Verification items for the finished model (mm, model axes). A direction names the side the tool comes from. Coordinates: 2 decimals unless noted, no trailing zeros. Order: outer loops, then holes, each group sorted by start corner. A loop starts at its lowest first (then second) coordinate and runs counter-clockwise, first axis right, second up. Notation, with made-up numbers: M 43.5,42 L 50.5,42 A8 ccw 50.5,51 Z; hole C 52.5,-11.5 d5. An arc over 180 degrees is marked long. Answer as a JSON object with one key per item and string values. Group by question number.
(1) Cross-section at A-A (z = 0). Count the separate pieces of the cut face and the enclosed holes in it, plus the area to 3 significant figures.
(2) Mould release check, pull along Z, two halves, no side actions. Record for faces 6 (the face through (1.99, -57.15, 0.84)), 7 (the face through (0, -22, 16)), 8 (the face through (2.15, 0.84, -56.99)): released by +Z, released by -Z, zero draft, split by the parting line, or undercut.
(3) Gauge pin test, flat ends, axial feed: pin 1 Ø3 at (x, y) = (-10.5, -2) entering from +Z; pin 2 Ø10 at (x, z) = (-11, -3.5) entering from +Y; pin 3 Ø3 at (x, y) = (-1.5, 25) entering from +Z; pin 4 Ø2 at (x, z) = (-4, -9) entering from -Y. Record the tip position at first contact, or that the pin passes through.
(4) Cross-section at C-C (x = -21.5). Enter the section's corners in (y, z), plus the area to 3 significant figures.
(5) Material ranges on line 1 (X direction, y = 31, z = -15); line 2 (Y direction, x = -4.5, z = -39); line 3 (Z direction, x = -1.75, y = 25), recorded low to high.
(6) Access from +Z, -Z, +X, -X, +Y, -Y to the whole of each face (thin tool, end or side, straight path). Record for faces 1 (the face through (-15, 28.333, 0)), 2 (the face through (-10, 0, 10)), 3 (the face through (0, 22, -16)), 4 (the face through (0, 29.333, 0)), 5 (the face through (-10, 0, -10)).
from build123d import *

# Parameters (mm, degrees)
SKETCH2_W           = 120
SKETCH2_H           = 120
BOSS_EXTRUDE1_DEPTH = 5
FILLET1_R           = 10
BOSS_EXTRUDE2_DEPTH = 50
SKETCH3_W           = 12.5
SKETCH3_H           = 30
CUT_EXTRUDE1_DEPTH  = 91
SKETCH5_W           = 14.5
SKETCH5_H           = 32
CUT_EXTRUDE2_DEPTH  = 10


with BuildPart() as part:
    # Sketch2 → Boss-Extrude1 (new, symmetric)
    with BuildSketch(Plane.YZ):
        Rectangle(SKETCH2_W, SKETCH2_H)
    extrude(amount=BOSS_EXTRUDE1_DEPTH, both=True)

    # Fillet1
    fillet1_edges = [part.edges().sort_by_distance(p)[0] for p in [
        (5, 60, 0),
        (5, 0, -60),
        (5, -60, 0),
        (5, 0, 60),
    ]]
    fillet(fillet1_edges, radius=FILLET1_R - 0.0001)  # a hair under: the kernel refuses the full size

    # Sketch4 → Boss-Extrude2 (add, symmetric)
    with BuildSketch(Plane(origin=(0, 0, 0), x_dir=(-1, 0, 0), z_dir=(0, 1, 0))):
        with BuildLine():
            Line((15, 10), (5, 10))
            Line((5, 10), (5, -10))
            Line((5, -10), (15, -10))
            ThreePointArc((15, -10), (25, 0), (15, 10))
        make_face()
    extrude(amount=BOSS_EXTRUDE2_DEPTH, both=True)

    # Sketch3 → Cut-Extrude1 (cut, through all)
    with BuildSketch(Plane.YZ.offset(5)):
        with Locations((-22.083333333, 0)):
            Rectangle(SKETCH3_W, SKETCH3_H)
        with Locations((22.083333333, 0)):
            Rectangle(SKETCH3_W, SKETCH3_H)
    extrude(amount=-CUT_EXTRUDE1_DEPTH, mode=Mode.SUBTRACT)

    # Sketch5 → Cut-Extrude2 (cut)
    with BuildSketch(Plane.YZ.offset(5)):
        with Locations((22.083333333, 0)):
            Rectangle(SKETCH5_W, SKETCH5_H)
        with Locations((-22.083333333, 0)):
            Rectangle(SKETCH5_W, SKETCH5_H)
    extrude(amount=-CUT_EXTRUDE2_DEPTH, mode=Mode.SUBTRACT)


solid = part.part
Taken from the geometry:
{
 "1": {"separate pieces": "3", "enclosed holes": "0", "area": "2,370 mm²"},
 "2": {"face 6": "zero draft", "face 7": "undercut", "face 8": "released by -Z"},
 "3": {"pin 1": "stops at z = 10", "pin 2": "stops at y = 50", "pin 3": "stops at z = 59.8", "pin 4": "stops at y = -60"},
 "4": {"outline": "M -50,-7.6 L -28.33,-7.6 L -28.33,7.6 L -50,7.6 Z; M -15.83,-7.6 L 15.83,-7.6 L 15.83,7.6 L -15.83,7.6 Z; M 28.33,-7.6 L 50,-7.6 L 50,7.6 L 28.33,7.6 Z", "area": "1,140 mm²"},
 "5": {"line 1": "x = -5 to 5", "line 2": "y = -59.99 to 59.99", "line 3": "z = -59.46 to -16, 16 to 59.46"},
 "6": {"face 1": "+Z, -Z, +X, -X", "face 2": "+Z, -X, +Y, -Y", "face 3": "+X, -X", "face 4": "+X", "face 5": "-Z, -X, +Y, -Y"}
}
